Geometry: see drawing. Coordinates: mm, zero at the bounding-box minimum. Give positions to 0.01 mm unless a question says otherwise; leave off trailing zeros. Write each loop counter-clockwise with the first axis right and the second up, starting at its lowest first coordinate (ties: lowest second). Pieces come first, ordered by that corner, then holes. Notation, with made-up numbers: (-36, 61.25) -> (-26, 61.25) arc R10 cw to (-26, 65.25) -> close; hole circle Ø10 at (58, -34). An arc over 180 degrees is marked (long way). Answer as a JSON object with one key per item and string values. Group by question number.
Item 1: Section query D-D on y = 31. Return the cut outline in (x, z), plus the area to 3 significant figures.
Item 2: Ray query, probe 1 along Y at (x, z) = (0.75, 35); probe 2 along Z at (x, y) = (1.4, 35); probe 3 along Y at (x, z) = (2.3, 49). Return the intervals inside material, ascending. Write a range as from..to.
Item 3: Section query B-B on z = 49. Return the cut outline in (x, y), plus the area to 3 significant figures.
Item 4: Section query A-A on z = 17. Return the cut outline in (x, y), plus the area to 3 significant figures.
Item 5: First-contact query: pin 1 Ø1.5 at (x, z) = (1.5, 51) entering from -Y; pin 2 Ø1.5 at (x, z) = (2, 16.5) entering from +Y; pin 3 Ø2.5 at (y, z) = (56, 35) entering from -X. Flat tips, straight axial feed; report the tip coordinate or a pass-through.
Item 6: Section query C-C on x = 0.95. Return the cut outline in (y, z), plus the area to 3 significant figures.
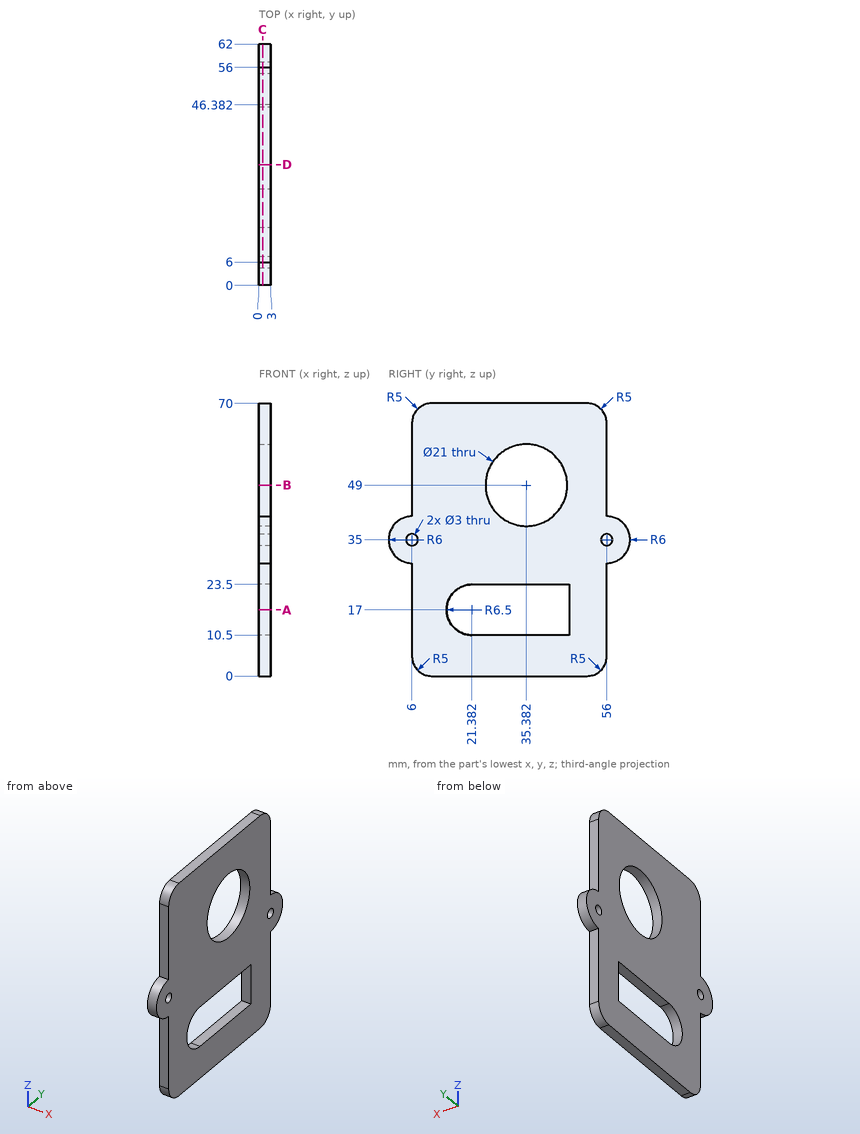
Worked answers:
{
 "1": {"outline": "(0, 0) -> (3, 0) -> (3, 10.5) -> (0, 10.5) -> close; (0, 23.5) -> (3, 23.5) -> (3, 39.46) -> (0, 39.46) -> close; (0, 58.54) -> (3, 58.54) -> (3, 70) -> (0, 70) -> close", "area": "114 mm^2"},
 "2": {"probe 1": "0..4.5, 7.5..54.5, 57.5..62", "probe 2": "0..10.5, 23.5..38.51, 59.49..70", "probe 3": "6..24.88, 45.88..56"},
 "3": {"outline": "(0, 6) -> (3, 6) -> (3, 24.88) -> (0, 24.88) -> close; (0, 45.88) -> (3, 45.88) -> (3, 56) -> (0, 56) -> close", "area": "87.0 mm^2"},
 "4": {"outline": "(0, 6) -> (3, 6) -> (3, 14.88) -> (0, 14.88) -> close; (0, 46.38) -> (3, 46.38) -> (3, 56) -> (0, 56) -> close", "area": "55.5 mm^2"},
 "5": {"pin 1": "y = 6", "pin 2": "y = 56", "pin 3": "through"},
 "6": {"outline": "(6, 5) arc R5 ccw to (11, 0) -> (51, 0) arc R5 ccw to (56, 5) -> (56, 29) arc R6 ccw to (56, 41) -> (56, 65) arc R5 ccw to (51, 70) -> (11, 70) arc R5 ccw to (6, 65) -> (6, 41) arc R6 ccw to (6, 29) -> close; hole circle Ø3 at (6, 35); hole (21.38, 10.5) -> (46.38, 10.5) -> (46.38, 23.5) -> (21.38, 23.5) arc R6.5 ccw to start; hole circle Ø21 at (35.38, 49); hole circle Ø3 at (56, 35)", "area": "2,840 mm^2"}
}
